Design review of the part built by this model. Coordinates are the model's own, in mm. Coordinates: 2 decimals unless noted, no trailing zeros. Answer as a JSON object with one key per item and string values. Group by question number.
1. Insertion check: pin 1 (0.7 mm diameter, centred on x = 4.5, y = -2.5, fed in from +Z). The pin has a flat end and moves straight along its axis. Give the tip position at first contact, or say it passes through.
2. Draft analysis for pull direction X (two halves, no side actions). For faces 1 (the flat face through (-5.08, -2, 0)), 2 (the flat face through (4, -2, 0)), 3 (the flat face through (5.08, -2, -1)), state which applies: +X half, -X half, draft (parallel to the pull), parting line (faces both ways), or undercut.
3. To check wall thickness, follow probe 1 along Z at (x, y) = (2.75, -3.4); probe 2 along X at (y, z) = (-0.7, 1.9); probe 3 along Z at (x, y) = (4.5, -0.55). State the ranges of each line that lie inside material, in increasing order.
from build123d import *

# Parameters (mm, degrees)
F1_DEPTH = 3.81


with BuildPart() as f1:
    # F0 (on Front) → F1 (new body)
    with BuildSketch(Plane.XZ):
        with BuildLine():
            Line((-5.08, 0), (-5.08, -2.54))
            Line((-5.08, -2.54), (5.08, -2.54))
            Line((5.08, -2.54), (5.08, 0))
            Line((5.08, 0), (3.6488212645, 0))
            add(Edge.make_bspline(
                [(0, 2.54), (0.9258067301, 2.1494416055), (2.5770675473, 1.4528449754), (3.3216856434, 0.4434575874), (3.6488212645, 0)],
                knots=[0, 0, 0, 0, 0.5606665022, 1, 1, 1, 1], degree=3))
            Line((0, 2.54), (-5.08, 2.54))
            Line((-5.08, 2.54), (-5.08, 0))
        make_face()
    extrude(amount=F1_DEPTH)


solid = f1.part
Findings below:
{
 "1": {"pin 1": "stops at z = 0"},
 "2": {"face 1": "-X half", "face 2": "draft", "face 3": "+X half"},
 "3": {"probe 1": "z = -2.54 to 1.06", "probe 2": "x = -5.08 to 1.44", "probe 3": "z = -2.54 to 0"}
}
